Model file for the job. Use its own axes, mm. A direction names the side the tool comes from. Round coordinates to 2 decimals unless told otherwise and drop trailing zeros. Loops run counter-clockwise (first coordinate to the right, second up) from the corner with the lowest first, then second, coordinate; pieces in that order, holes last.
from build123d import *

# Parameters (mm, degrees)
SKETCH1_R               = 3.15
BOSS_EXTRUDE1_DEPTH     = 31.75
SKETCH4_W               = 8.89
SKETCH4_H               = 21.59
CUT_EXTRUDE1_DEPTH      = 41.902084605
SKETCH2_R               = 1.25
CUT_EXTRUDE2_DEPTH      = 2.54
SKETCH5_W               = 21.59
SKETCH5_H               = 8.89
CUT_EXTRUDE3_DEPTH      = 50.285164096
SKETCH6_R               = 1.75
CUT_EXTRUDE4_DEPTH      = 2.54
CUT_EXTRUDE5_REACH      = 81.487
CUT_EXTRUDE5_END_RADIUS = 3.15
SKETCH7_R               = 1.95
CUT_EXTRUDE6_DEPTH      = 6.35


with BuildPart() as part:
    # Sketch1 → Boss-Extrude1 (new body)
    with BuildSketch(Plane(origin=(0, 0, 0), x_dir=(0, 0, -1), z_dir=(1, 0, 0))):
        with BuildLine():
            Line((20.32, 15.875), (0, 15.875))
            ThreePointArc((0, 15.875), (-15.875, 0), (0, -15.875))
            Line((0, -15.875), (20.32, -15.875))
            Line((20.32, -15.875), (20.32, 15.875))
        make_face()
        Circle(SKETCH1_R, mode=Mode.SUBTRACT)
    extrude(amount=BOSS_EXTRUDE1_DEPTH)

    # Sketch4 → Cut-Extrude1 (cut, through all)
    with BuildSketch(Plane.ZY):
        with Locations((-13.335, 0)):
            Rectangle(SKETCH4_W, SKETCH4_H)
    extrude(amount=-CUT_EXTRUDE1_DEPTH, mode=Mode.SUBTRACT)

    # Sketch2 → Cut-Extrude2 (cut)
    with BuildSketch(Plane(origin=(0, 0, -20.32), x_dir=(-1, 0, 0), z_dir=(0, 0, -1))):
        with Locations((-26.035, 6.35)):
            Circle(SKETCH2_R)
        with Locations((-5.715, 6.35)):
            Circle(SKETCH2_R)
        with Locations((-5.715, -6.35)):
            Circle(SKETCH2_R)
        with Locations((-26.035, -6.35)):
            Circle(SKETCH2_R)
    extrude(amount=-CUT_EXTRUDE2_DEPTH, mode=Mode.SUBTRACT)

    # Sketch5 → Cut-Extrude3 (cut, through all)
    with BuildSketch(Plane(origin=(0, 15.875, 0), x_dir=(1, 0, 0), z_dir=(0, 1, 0))):
        with Locations((15.875, 13.335)):
            Rectangle(SKETCH5_W, SKETCH5_H)
    extrude(amount=-CUT_EXTRUDE3_DEPTH, mode=Mode.SUBTRACT)

    # Sketch6 → Cut-Extrude4 (cut)
    with BuildSketch(Plane(origin=(0, 0, -20.32), x_dir=(-1, 0, 0), z_dir=(0, 0, -1))):
        with Locations((-15.875, 12.7)):
            Circle(SKETCH6_R)
        with Locations((-15.875, -12.7)):
            Circle(SKETCH6_R)
    extrude(amount=-CUT_EXTRUDE4_DEPTH, mode=Mode.SUBTRACT)

    # Cut-Extrude5: up to this cylinder (the profile starts outside it)
    cut_extrude5_end = Plane(origin=(15.875, 0, 0), z_dir=(-1, 0, 0)) * Cylinder(CUT_EXTRUDE5_END_RADIUS, 170.274, mode=Mode.PRIVATE)
    # Sketch7 → Cut-Extrude5 (cut, up to the surface)
    with BuildSketch(Plane.XY.offset(50.8), mode=Mode.PRIVATE) as cut_extrude5_sk1:
        with Locations((15.875, 0)):
            Circle(SKETCH7_R)
    cut_extrude5_tool1 = extrude(cut_extrude5_sk1.sketch, amount=-CUT_EXTRUDE5_REACH, mode=Mode.PRIVATE) - cut_extrude5_end
    add(cut_extrude5_tool1.solids().sort_by_distance((15.875, 0, 50.8))[0], mode=Mode.SUBTRACT)

    # Sketch8 → Cut-Extrude6 (cut)
    with BuildSketch(Plane(origin=(0, 0, -8.89), x_dir=(-1, 0, 0), z_dir=(0, 0, -1))):
        Polygon((-26.67, 9.525), (-5.08, 9.525), (-5.08, 10.795), (-5.08, 15.875), (-26.67, 15.875), (-26.67, 10.795), align=None)
        Polygon((-26.67, -9.525), (-5.08, -9.525), (-5.08, -10.795), (-5.08, -15.875), (-26.67, -15.875), (-26.67, -10.795), align=None)
    extrude(amount=-CUT_EXTRUDE6_DEPTH, mode=Mode.SUBTRACT)


solid = part.part
Q1. Slice it at C-C on y = 12.7. Give the cut face in (x, z) (3 decimals).
Q2. Pull direction X, two halves, no side cores. Call faces 1 (the face through (3, -10.795, -13)), 2 (the face through (0, 4, -2)), 3 (the face through (31.75, 4, -2)), 4 (the face through (5.88, 7.59, -19.07)): pulls with the +X half, pulls with the -X half, needs draft (parallel to the pull), parting line crosses it, or undercut.
Q3. Probe line 1 (Z direction, x = 23, y = 0) (3 decimals); line 2 (X direction, y = 10, z = -7); line 3 (X direction, y = -7, z = -19). List the from-to ranges inside material, lowest first.
Q4. Tool access for faces 5 (the face through (16, 0, -17.78)), 6 (the face through (13.927, 0.086, 9.27)), 7 (the face through (16, -9.525, -6)), 8 (the face through (5.08, 13, -10)): list every direction of +Z, -Z, +X, -X, +Y, -Y with a clear straight run to the whole face (end or side of a thin tool).
Q5. Slice it at D-D on z = -0.5. Give the cut face in (x, y) (3 decimals).
Q6. Slice it at B-B on x = 21. Give the cut face in (y, z) (3 decimals).
Q7. Slice it at A-A on z = -9.5. Give the cut face in (x, y) (3 decimals).
Q8. Flat gauge pins, fed straight in: P1, Ø4, axis at x = 15, z = 5.5, coming from the +Y side; P2, Ø1.5, axis at x = 26.035, y = -6.35, coming from the -Z side; P3, Ø3, axis at x = 5.715, y = -6.35, coming from the +Z side. Where does each tip first touch, or does it go through?
Reply:
1. outline: (0, -20.32) - (14.125, -20.32) - (14.125, -17.78) - (5.08, -17.78) - (5.08, -2.54) - (26.67, -2.54) - (26.67, -17.78) - (17.625, -17.78) - (17.625, -20.32) - (31.75, -20.32) - (31.75, 9.525) - (0, 9.525) - close
2. face 1: needs draft
2. face 2: pulls with the -X half
2. face 3: pulls with the +X half
2. face 4: undercut
3. line 1: z = -20.32 to -17.78, -8.89 to -3.15, 3.15 to 15.875
3. line 2: x = 0 to 5.08, 26.67 to 31.75
3. line 3: x = 0 to 4.65, 6.78 to 24.97, 27.1 to 31.75
4. face 5: none
4. face 6: +Z
4. face 7: -Y
4. face 8: +Y
5. outline: (0, -15.875) - (31.75, -15.875) - (31.75, -3.11) - (0, -3.11) - close; (0, 3.11) - (31.75, 3.11) - (31.75, 15.875) - (0, 15.875) - close
6. outline: (-15.875, -20.32) - (15.875, -20.32) - (15.875, -17.78) - (-15.875, -17.78) - close; (-15.875, -2.54) - (-9.525, -2.54) - (-9.525, -8.89) - (9.525, -8.89) - (9.525, -2.54) - (15.875, -2.54) - (15.875, 0) arc R15.875 ccw to (-15.875, 0) - close; hole circle Ø6.3 at (0, 0)
7. outline: (0, -15.875) - (5.08, -15.875) - (5.08, -10.795) - (0, -10.795) - close; (0, 10.795) - (5.08, 10.795) - (5.08, 15.875) - (0, 15.875) - close; (26.67, -15.875) - (31.75, -15.875) - (31.75, -10.795) - (26.67, -10.795) - close; (26.67, 10.795) - (31.75, 10.795) - (31.75, 15.875) - (26.67, 15.875) - close
8. P1: stops at y = 15.48
8. P2: stops at z = -8.89
8. P3: stops at z = 15.12
